The model under review builds one solid part; all positions refer to its coordinate system, in mm. A direction names the side the tool comes from. Round coordinates to 2 decimals unless told otherwise and drop trailing zeros. Loops run counter-clockwise (first coordinate to the right, second up) from the corner with the lowest first, then second, coordinate; pieces in that order, holes last. Notation, with made-up numbers: (51, 69) -> (77, 69) arc R22 cw to (77, 100) -> close; hole circle Ø1 at (-38, -27). An arc over 180 degrees is marked (long way). Use CSV: the item, a comma, the result in double quotes. Start each with the question number.
```python
from build123d import *

# Parameters (mm, degrees)
CYLINDER008_R             = 1.65
CYLINDER008_DEPTH         = 10
BOX_W                     = 15
BOX_H                     = 3
BOX_DEPTH                 = 10
CYLINDER014_R             = 7.25
CYLINDER014_DEPTH         = 1
CYLINDER013_R             = 6.5
CYLINDER013_DEPTH         = 32
FUSION010_PLACEMENT_ANGLE = 90
CYLINDER010_R             = 3.25
CYLINDER010_DEPTH         = 10
CYLINDER009_R             = 5.5
CYLINDER009_DEPTH         = 6
CYLINDER012_R             = 3.25
CYLINDER012_DEPTH         = 10
CYLINDER011_R             = 5.5
CYLINDER011_DEPTH         = 6
BOX006_W                  = 15
BOX006_H                  = 20
BOX006_DEPTH              = 20
BOX005_W                  = 15
BOX005_H                  = 20
BOX005_DEPTH              = 20
BOX004_W                  = 15
BOX004_H                  = 63
BOX004_DEPTH              = 15


with BuildPart() as m4wormscrew:
    # Cylinder008 → Cylinder008 (new body)
    with BuildSketch(Plane(origin=(0, -3, 12.5), x_dir=(1, 0, 0), z_dir=(0, -1, 0))):
        Circle(CYLINDER008_R)
    extrude(amount=CYLINDER008_DEPTH)


with BuildPart() as cube:
    # Box → Box (new body)
    with BuildSketch(Plane(origin=(-7.5, -1.5, 9), x_dir=(1, 0, 0), z_dir=(0, 0, 1))):
        with Locations((7.5, 1.5)):
            Rectangle(BOX_W, BOX_H)
    extrude(amount=BOX_DEPTH)


with BuildPart() as cylinder014:
    # Cylinder014 → Cylinder014 (new body)
    with BuildSketch(Plane.XY):
        Circle(CYLINDER014_R)
    extrude(amount=CYLINDER014_DEPTH)


with BuildPart() as lasermoduletemplate002:
    # Cylinder013 → Cylinder013 (new body)
    with BuildSketch(Plane.XY):
        Circle(CYLINDER013_R)
    extrude(amount=CYLINDER013_DEPTH)

    # Fusion010: union Cylinder014
    add(cylinder014.part)


with BuildPart() as lasermoduletemplate002_1:
    # Fusion010 placement: moved
    add(lasermoduletemplate002.part.moved(Location((-7.5, 0, 7.5))).rotate(Axis((-7.5, 0, 7.5), (0, 1, 0)), FUSION010_PLACEMENT_ANGLE))


with BuildPart() as cylinder010:
    # Cylinder010 → Cylinder010 (new body)
    with BuildSketch(Plane.XY):
        Circle(CYLINDER010_R)
    extrude(amount=CYLINDER010_DEPTH)


with BuildPart() as screwthrough003:
    # Cylinder009 → Cylinder009 (new body)
    with BuildSketch(Plane.XY.offset(4)):
        Circle(CYLINDER009_R)
    extrude(amount=CYLINDER009_DEPTH)

    # Fusion007: union Cylinder010
    add(cylinder010.part)


with BuildPart() as screwthrough003_1:
    # Fusion007 placement: moved
    add(screwthrough003.part.moved(Location((0, -21.5, 0))))


with BuildPart() as cylinder012:
    # Cylinder012 → Cylinder012 (new body)
    with BuildSketch(Plane.XY):
        Circle(CYLINDER012_R)
    extrude(amount=CYLINDER012_DEPTH)


with BuildPart() as fusion009:
    # Cylinder011 → Cylinder011 (new body)
    with BuildSketch(Plane.XY.offset(4)):
        Circle(CYLINDER011_R)
    extrude(amount=CYLINDER011_DEPTH)

    # Fusion008: union Cylinder012
    add(cylinder012.part)


with BuildPart() as fusion009_1:
    # Fusion008 placement: moved
    add(fusion009.part.moved(Location((0, 21.5, 0))))

    # Fusion009: union ScrewThrough003
    add(screwthrough003_1.part)


with BuildPart() as cube006:
    # Box006 → Box006 (new body)
    with BuildSketch(Plane(origin=(-15, -31.5, 10), x_dir=(1, 0, 0), z_dir=(0, 0, 1))):
        with Locations((7.5, 10)):
            Rectangle(BOX006_W, BOX006_H)
    extrude(amount=BOX006_DEPTH)


with BuildPart() as fusion006:
    # Box005 → Box005 (new body)
    with BuildSketch(Plane(origin=(-15, 11.5, 10), x_dir=(1, 0, 0), z_dir=(0, 0, 1))):
        with Locations((7.5, 10)):
            Rectangle(BOX005_W, BOX005_H)
    extrude(amount=BOX005_DEPTH)

    # Fusion006: union Cube006
    add(cube006.part)


with BuildPart() as cut008:
    # Box004 → Box004 (new body)
    with BuildSketch(Plane(origin=(-15, -31.5, 0), x_dir=(1, 0, 0), z_dir=(0, 0, 1))):
        with Locations((7.5, 31.5)):
            Rectangle(BOX004_W, BOX004_H)
    extrude(amount=BOX004_DEPTH)

    # Cut005: cut Fusion006
    add(fusion006.part, mode=Mode.SUBTRACT)


with BuildPart() as cut008_1:
    # Cut005 placement: moved
    add(cut008.part.moved(Location((7.5, 0, 0))))

    # Cut006: cut Fusion009
    add(fusion009_1.part, mode=Mode.SUBTRACT)

    # Cut007: cut LaserModuleTemplate002
    add(lasermoduletemplate002_1.part, mode=Mode.SUBTRACT)

    # Cut: cut Cube
    add(cube.part, mode=Mode.SUBTRACT)

    # Cut008: cut M4WormScrew
    add(m4wormscrew.part, mode=Mode.SUBTRACT)


solid = cut008_1.part
```
1. Take a section at D-D, the plane z = 12.5. Give the boundary of the cut face in (x, y).
2. Clearance check with flat-ended pins moving along their axes: P1, Ø8.5, axis at y = 0, z = 7.5, coming from the -X side; P2, Ø5.5, axis at x = 0.5, y = 19, coming from the +Z side; P3, Ø4.5, axis at x = 1.5, y = -18.5, coming from the +Z side; P4, Ø1, axis at x = 0.5, z = 14, coming from the -Y side. State where each tip first meets the part, or that it passes through.
3. Take a section at A-A, the plane z = 7.5. Give the boundary of the cut face in (x, y), then the cut area to 3 significant figures.
4. Take a section at B-B, the plane y = -21.5. Give the boundary of the cut face in (x, z).
5. The part is to be moulded in two halves that separate along X. For faces 1 (the face through (7.5, -0.4, 0.7)), 2 (the face through (0, -31.5, 5)), 3 (the face through (1.75, -18.76, 1.97)), say which applies: pulls with the +X half, pulls with the -X half, needs draft (parallel to the pull), parting line crosses it, or undercut.
6. For line 1 along Y through (x, z) = (3, 7.5); line 2 along Y through (x, z) = (-3.5, 5.75); line 3 along Z through (x, y) = (4.5, -27.5), list the stretches that pass through material, from the lowest coordinate up. Write a range as from..to.
7. Take a section at C-C, the plane x = 0. Count the separate pieces of the cut face and the enclosed holes in it, then the cut area to 3 significant figures.
8. For faces 4 (the face through (-3.4, -16.9, 10)), 5 (the face through (-6.5, 4, 2)), 6 (the face through (0, 1.5, 14)), 7 (the face through (-0.716, 26.953, 6.958)), list the 3-axis set-ups (+Z, -Z, +X, -X, +Y, -Y) from which the entire face can be reached by the end or side of a thin tool; tool diameter is ignored.
Results:
1,outline,"(-7.5, -11.5) -> (-1.65, -11.5) -> (-1.65, -4.15) -> (-6.5, -4.15) -> (-6.5, -5.25) -> (-7.5, -5.25) -> close; (-7.5, 5.25) -> (-6.5, 5.25) -> (-6.5, 4.15) -> (7.5, 4.15) -> (7.5, 11.5) -> (-7.5, 11.5) -> close; (1.65, -11.5) -> (7.5, -11.5) -> (7.5, -4.15) -> (1.65, -4.15) -> close"
2,P1,"through"
2,P2,"z = 4"
2,P3,"z = 10"
2,P4,"y = -11.5"
3,outline,"(-7.5, -31.5) -> (7.5, -31.5) -> (7.5, -6.5) -> (-6.5, -6.5) -> (-6.5, -7.25) -> (-7.5, -7.25) -> close; (-7.5, 7.25) -> (-6.5, 7.25) -> (-6.5, 6.5) -> (7.5, 6.5) -> (7.5, 31.5) -> (-7.5, 31.5) -> close; hole circle Ø11 at (0, -21.5); hole circle Ø11 at (0, 21.5)"
3,area,"558 mm²"
4,outline,"(-7.5, 0) -> (-3.25, 0) -> (-3.25, 4) -> (-5.5, 4) -> (-5.5, 10) -> (-7.5, 10) -> close; (3.25, 0) -> (7.5, 0) -> (7.5, 10) -> (5.5, 10) -> (5.5, 4) -> (3.25, 4) -> close"
5,face 1,"pulls with the +X half"
5,face 2,"needs draft"
5,face 3,"undercut"
6,line 1,"-31.5..-26.11, -16.89..-6.5, 6.5..16.89, 26.11..31.5"
6,line 2,"-31.5..-25.74, -17.26..-6.26, 6.26..17.26, 25.74..31.5"
6,line 3,"0..10"
7,separate pieces,"4"
7,enclosed holes,"0"
7,area,"401 mm²"
8,face 4,"+Z, +X, -X, -Y"
8,face 5,"-X"
8,face 6,"+Z, +X, -X"
8,face 7,"+Z"
